from build123d import *

# Parameters (mm, degrees)
F1_DEPTH = 5
F3_DEPTH = 5


with BuildPart() as f1:
    # F0 (on Front) → F1 (new body)
    with BuildSketch(Plane.XZ):
        with BuildLine():
            ThreePointArc((-0.487665, 2.196516), (-1.408058, -1.754957), (2.25, 0))
            ThreePointArc((2.25, 0), (1.754957, 1.408058), (0.487665, 2.196516))
            ThreePointArc((0.487665, 2.196516), (0, 2.25), (-0.487665, 2.196516))
        make_face()
    extrude(amount=F1_DEPTH)

    # F2 (on Front) + F0 (on Front) → F3 (join)
    with BuildSketch(Plane.XZ):
        with BuildLine():
            ThreePointArc((-1.685609, 1.490377), (-1.322517, 1.820288), (-0.896551, 2.063661))
            ThreePointArc((-0.896551, 2.063661), (-1.286731, 2.661442), (-1.865962, 3.078666))
            ThreePointArc((-1.865962, 3.078666), (-2.116027, 2.912461), (-2.351372, 2.725995))
            ThreePointArc((-2.351372, 2.725995), (-2.13356, 2.046185), (-1.685609, 1.490377))
        make_face()
        with BuildLine():
            ThreePointArc((0.896551, 2.063661), (1.322517, 1.820288), (1.685609, 1.490377))
            ThreePointArc((1.685609, 1.490377), (2.13356, 2.046185), (2.351372, 2.725995))
            ThreePointArc((2.351372, 2.725995), (2.116027, 2.912461), (1.865962, 3.078666))
            ThreePointArc((1.865962, 3.078666), (1.286731, 2.661442), (0.896551, 2.063661))
        make_face()
        with BuildLine():
            ThreePointArc((1.938314, 1.142558), (2.139877, 0.695288), (2.239708, 0.214964))
            ThreePointArc((2.239708, 0.214964), (2.928804, 0.401323), (3.5046, 0.823275))
            ThreePointArc((3.5046, 0.823275), (3.423803, 1.112461), (3.319189, 1.393909))
            ThreePointArc((3.319189, 1.393909), (2.605344, 1.39683), (1.938314, 1.142558))
        make_face()
        with BuildLine():
            ThreePointArc((3.5046, -0.823275), (2.928804, -0.401323), (2.239708, -0.214964))
            ThreePointArc((2.239708, -0.214964), (2.139877, -0.695288), (1.938314, -1.142558))
            ThreePointArc((1.938314, -1.142558), (2.605344, -1.39683), (3.319189, -1.393909))
            ThreePointArc((3.319189, -1.393909), (3.423803, -1.112461), (3.5046, -0.823275))
        make_face()
        with BuildLine():
            ThreePointArc((2.351372, -2.725995), (2.13356, -2.046185), (1.685609, -1.490377))
            ThreePointArc((1.685609, -1.490377), (1.322517, -1.820288), (0.896551, -2.063661))
            ThreePointArc((0.896551, -2.063661), (1.286731, -2.661442), (1.865962, -3.078666))
            ThreePointArc((1.865962, -3.078666), (2.116027, -2.912461), (2.351372, -2.725995))
        make_face()
        with BuildLine():
            ThreePointArc((0.3, -3.587478), (0.523369, -2.909474), (0.487665, -2.196516))
            ThreePointArc((0.487665, -2.196516), (0, -2.25), (-0.487665, -2.196516))
            ThreePointArc((-0.487665, -2.196516), (-0.523369, -2.909474), (-0.3, -3.587478))
            ThreePointArc((-0.3, -3.587478), (0, -3.6), (0.3, -3.587478))
        make_face()
        with BuildLine():
            ThreePointArc((-2.239708, 0.214964), (-2.139877, 0.695288), (-1.938314, 1.142558))
            ThreePointArc((-1.938314, 1.142558), (-2.605344, 1.39683), (-3.319189, 1.393909))
            ThreePointArc((-3.319189, 1.393909), (-3.423803, 1.112461), (-3.5046, 0.823275))
            ThreePointArc((-3.5046, 0.823275), (-2.928804, 0.401323), (-2.239708, 0.214964))
        make_face()
        with BuildLine():
            ThreePointArc((-1.865962, -3.078666), (-1.286731, -2.661442), (-0.896551, -2.063661))
            ThreePointArc((-0.896551, -2.063661), (-1.322517, -1.820288), (-1.685609, -1.490377))
            ThreePointArc((-1.685609, -1.490377), (-2.13356, -2.046185), (-2.351372, -2.725995))
            ThreePointArc((-2.351372, -2.725995), (-2.116027, -2.912461), (-1.865962, -3.078666))
        make_face()
        with BuildLine():
            ThreePointArc((-3.319189, -1.393909), (-2.605344, -1.39683), (-1.938314, -1.142558))
            ThreePointArc((-1.938314, -1.142558), (-2.139877, -0.695288), (-2.239708, -0.214964))
            ThreePointArc((-2.239708, -0.214964), (-2.928804, -0.401323), (-3.5046, -0.823275))
            ThreePointArc((-3.5046, -0.823275), (-3.423803, -1.112461), (-3.319189, -1.393909))
        make_face()
    with BuildSketch(Plane.XZ):
        with BuildLine():
            ThreePointArc((-0.487665, 2.196516), (0, 2.25), (0.487665, 2.196516))
            ThreePointArc((0.487665, 2.196516), (0.523369, 2.909474), (0.3, 3.587478))
            ThreePointArc((0.3, 3.587478), (0, 3.6), (-0.3, 3.587478))
            ThreePointArc((-0.3, 3.587478), (-0.523369, 2.909474), (-0.487665, 2.196516))
        make_face()
    extrude(amount=F3_DEPTH)


solid = f1.part
Can you work these out from the model? Positions are in its coordinate system, mm. A direction names the side the tool comes from. Give positions to 0.01 mm unless a question says otherwise; leave off trailing zeros. Loops run counter-clockwise (first coordinate to the right, second up) from the corner with the lowest first, then second, coordinate; pieces in that order, holes last. Notation, with made-up numbers: (-33, -10.5) - (-9, -10.5) arc R14 cw to (-9, 4.5) - close; hole circle Ø6 at (-6, 46). An arc over 180 degrees is marked (long way). Return JSON: item names as keys, results as strings.
1. I want a section at A-A on z = 2.5. Please give me the cut outline in (x, y).
Output values:
{"outline": "(-2.31, -5) - (-1.15, -5) - (-1.15, 0) - (-2.31, 0) - close; (-0.54, -5) - (0.54, -5) - (0.54, 0) - (-0.54, 0) - close; (1.15, -5) - (2.31, -5) - (2.31, 0) - (1.15, 0) - close"}
2. I want a section at C-C on x = -1.25. Please give me the cut outline in (y, z).
Output values:
{"outline": "(-5, -2.62) - (0, -2.62) - (0, 2.62) - (-5, 2.62) - close"}
3. If I drill on line 1 (X direction, y = -3.25, z = 2.25); line 2 (X direction, y = -0.95, z = 2.75); line 3 (Z direction, x = 3, y = -3.05), over which ranges is the centre line in solid material (lowest first)?
Output values:
{"line 1": "x = -2.23 to -0.99, -0.5 to 0.5, 0.99 to 2.23", "line 2": "x = -2.32 to -1.38, -0.54 to 0.54, 1.38 to 2.32", "line 3": "z = -1.43 to -0.44, 0.44 to 1.43"}
4. I'm going to push flat-ended pins straight in: pin 1 Ø1 at (x, y) = (-1.5, -1.5) entering from -Z; pin 2 Ø1 at (y, z) = (-3, -1.5) entering from -X. Where does each tip first touch, or does it pass through?
Output values:
{"pin 1": "stops at z = -3.08", "pin 2": "stops at x = -3.46"}
5. I want a section at B-B on x = -2.5. Please give me the cut outline in (y, z), and give its area (3 significant figures).
Output values:
{"outline": "(-5, -1.37) - (0, -1.37) - (0, -0.25) - (-5, -0.25) - close; (-5, 0.25) - (0, 0.25) - (0, 1.37) - (-5, 1.37) - close", "area": "11.2 mm²"}
6. We'd pull the mould along Z, two halves only. Please class faces 5 (the face through (1.294, -2.465, 2.669)), 6 (the face through (0.525, -2.465, 2.9)), 7 (the face through (-1.294, -2.465, -2.669)), 8 (the face through (0, -5, 0)): +Z half, -Z half, draft (parallel to the pull), parting line (faces both ways), or undercut.
Output values:
{"face 5": "+Z half", "face 6": "undercut", "face 7": "-Z half", "face 8": "draft"}
7. For faces 1 (the face through (2.62, -2.46, 1.4)), 2 (the face through (1.28, -2.465, -2.654)), 3 (the face through (-2.13, -2.46, -2.04)), 4 (the face through (2.14, -2.46, -2.06)), which set-ups out of +Z, -Z, +X, -X, +Y, -Y let a thin tool reach every point of the face, with its end or its side?
Output values:
{"face 1": "+Y, -Y", "face 2": "-Z, +Y, -Y", "face 3": "-X, +Y, -Y", "face 4": "+X, +Y, -Y"}
